Geometry check sheet. Reference: the model listing, model coordinates, mm. A direction names the side the tool comes from. Round coordinates to 2 decimals unless told otherwise and drop trailing zeros. Write each loop counter-clockwise with the first axis right and the second up, starting at its lowest first coordinate (ties: lowest second). Pieces come first, ordered by that corner, then holes. Notation, with made-up numbers: (-8.75, -3) - (10.25, -3) arc R22 ccw to (10.25, 22) - close; hole circle Ø3 at (-39.5, 3.5). An arc over 180 degrees is marked (long way). Return JSON: item names as keys, results as strings.
```python
from build123d import *

# Parameters (mm, degrees)
BOSS_EXTRUDE1_DEPTH = 25
SKETCH5_R           = 1.25
SKETCH5_R_2         = 11
CUT_EXTRUDE1_DEPTH  = 67.430584071
CUT_EXTRUDE2_DEPTH  = 77.502826745
CHAMFER1_SIZE       = 5


with BuildPart() as part:
    # Sketch4 → Boss-Extrude1 (new, symmetric)
    with BuildSketch(Plane(origin=(0, 0, 0), x_dir=(0, 0, -1), z_dir=(1, 0, 0))):
        with BuildLine():
            Line((0, 21.15), (0, -27.5))
            Line((0, -27.5), (50.85, -27.5))
            Line((50.85, -27.5), (50.85, -30.25))
            Line((50.85, -30.25), (0, -30.25))
            ThreePointArc((0, -30.25), (-1.944543648, -29.444543648), (-2.75, -27.5))
            Line((-2.75, -27.5), (-2.75, 21.15))
            Line((-2.75, 21.15), (0, 21.15))
        make_face()
    extrude(amount=BOSS_EXTRUDE1_DEPTH, both=True)

    # Sketch5 → Cut-Extrude1 (cut, through all)
    with BuildSketch(Plane.XY.offset(2.75)):
        with Locations((-15.5, -15.5)):
            Circle(SKETCH5_R)
        with Locations((-15.5, 15.5)):
            Circle(SKETCH5_R)
        with Locations((15.5, 15.5)):
            Circle(SKETCH5_R)
        with Locations((15.5, -15.5)):
            Circle(SKETCH5_R)
        Circle(SKETCH5_R_2)
    extrude(amount=-CUT_EXTRUDE1_DEPTH, mode=Mode.SUBTRACT)

    # Sketch6 → Cut-Extrude2 (cut, through all)
    with BuildSketch(Plane.XZ.offset(30.25)):
        with BuildLine():
            Line((-12.82, -9.995), (-12.82, -41.55))
            ThreePointArc((-12.82, -41.55), (-14.945, -43.675), (-17.07, -41.55))
            Line((-17.07, -41.55), (-17.07, -9.995))
            ThreePointArc((-17.07, -9.995), (-14.945, -7.87), (-12.82, -9.995))
        make_face()
        with BuildLine():
            Line((12.82, -9.995), (12.82, -41.55))
            ThreePointArc((12.82, -41.55), (14.945, -43.675), (17.07, -41.55))
            Line((17.07, -41.55), (17.07, -9.995))
            ThreePointArc((17.07, -9.995), (14.945, -7.87), (12.82, -9.995))
        make_face()
    extrude(amount=-CUT_EXTRUDE2_DEPTH, mode=Mode.SUBTRACT)

    # Chamfer1
    chamfer1_edges = [part.edges().sort_by_distance(p)[0] for p in [
        (25, -28.875, -50.85),
        (25, 21.15, 1.375),
        (-25, -28.875, -50.85),
        (-25, 21.15, 1.375),
    ]]
    chamfer(chamfer1_edges, length=CHAMFER1_SIZE)


solid = part.part
```
(1) Section check D-D, the plane x = -21. Enter the section's corners in (y, z).
Response values:
{"outline": "(-30.25, -49.85) - (-27.5, -49.85) - (-27.5, 0) - (20.15, 0) - (20.15, 2.75) - (-27.5, 2.75) arc R2.75 ccw to (-30.25, 0) - close"}
(2) Section check A-A, the plane y = -15.5. Enter the section's corners in (x, z), plus the area to 3 significant figures.
Response values:
{"outline": "(-25, 0) - (-16.75, 0) - (-16.75, 2.75) - (-25, 2.75) - close; (-14.25, 0) - (14.25, 0) - (14.25, 2.75) - (-14.25, 2.75) - close; (16.75, 0) - (25, 0) - (25, 2.75) - (16.75, 2.75) - close", "area": "124 mm^2"}
(3) Access from +Z, -Z, +X, -X, +Y, -Y to the whole of each face (thin tool, end or side, straight path). Record for faces 1 (the face through (0, -27.5, -25)), 2 (the face through (0, -14, 2.75)), 3 (the face through (14.898, -28.894, -43.674)).
Response values:
{"face 1": "-Z, +X, -X, +Y", "face 2": "+Z, +X, -X, +Y, -Y", "face 3": "+Y, -Y"}
(4) Gauge pin test, flat ends, axial feed: pin 1 (1.5 mm diameter, centred on x = -2.5, z = -33.5, fed in from +Y); pin 2 (10 mm diameter, centred on x = 14, z = -32, fed in from -Y). Record the tip position at first contact, or that the pin passes through.
Response values:
{"pin 1": "stops at y = -27.5", "pin 2": "stops at y = -30.25"}
(5) Section check C-C, the plane x = 4. Enter the section's corners in (y, z), plus the area to 3 significant figures.
Response values:
{"outline": "(-30.25, -50.85) - (-27.5, -50.85) - (-27.5, 0) - (-10.25, 0) - (-10.25, 2.75) - (-27.5, 2.75) arc R2.75 ccw to (-30.25, 0) - close; (10.25, 0) - (21.15, 0) - (21.15, 2.75) - (10.25, 2.75) - close", "area": "223 mm^2"}
(6) Section check B-B, the plane z = -22. Enter the section's corners in (x, y), plus the area to 3 significant figures.
Response values:
{"outline": "(-25, -30.25) - (-17.07, -30.25) - (-17.07, -27.5) - (-25, -27.5) - close; (-12.82, -30.25) - (12.82, -30.25) - (12.82, -27.5) - (-12.82, -27.5) - close; (17.07, -30.25) - (25, -30.25) - (25, -27.5) - (17.07, -27.5) - close", "area": "114 mm^2"}
(7) Material ranges on line 1 along Y through (x, z) = (15.5, 1.05); line 2 along Y through (x, z) = (15.5, 1.25); line 3 along Z through (x, y) = (-7, 15.5), recorded low to high. Write a range as [from, to].
Response values:
{"line 1": "y = [-30.04, -16.75], [-14.25, 14.25], [16.75, 21.15]", "line 2": "y = [-29.95, -16.75], [-14.25, 14.25], [16.75, 21.15]", "line 3": "z = [0, 2.75]"}
(8) Release check for a two-part mould opening along Z. For faces 4 (the face through (25, -28, -14)), 5 (the face through (0, -29, -50.85)), 6 (the face through (17.07, -29, -26)) record: pulls with the +Z half, pulls with the -Z half, needs draft (parallel to the pull), parting line crosses it, or undercut.
Response values:
{"face 4": "needs draft", "face 5": "pulls with the -Z half", "face 6": "undercut"}
